CAD build for the part. Positions are in the model's coordinates, mm. Face numbers are marked on the shaded views. A direction names the side the tool comes from. Coordinates: 2 decimals unless noted, no trailing zeros. Loops run counter-clockwise (first coordinate to the right, second up) from the corner with the lowest first, then second, coordinate; pieces in that order, holes last. Notation, with made-up numbers: (-2, 69.25) - (38, 69.25) arc R30 cw to (38, 102.25) - close; hole circle Ø6 at (44, 6). An arc over 180 degrees is marked (long way). Put each result on its own line as item: value.
```python
from build123d import *

# Parameters (mm, degrees)
SALIENTE_EXTRUIR1_DEPTH    = 14
CROQUIS2_W                 = 0.4
CROQUIS2_H                 = 0.4
CORTAR_EXTRUIR1_DEPTH      = 1
CORTAR_EXTRUIR1_DEPTH_BACK = 15
SALIENTE_EXTRUIR2_DEPTH    = 14
CORTAR_EXTRUIR2_DEPTH      = 1
CORTAR_EXTRUIR2_DEPTH_BACK = 5.5
CORTAR_EXTRUIR3_DEPTH      = 5.5
SALIENTE_EXTRUIR3_DEPTH    = 14
CROQUIS7_R                 = 1
CORTAR_EXTRUIR4_DEPTH      = 4
REDONDEO3_R                = 0.4
CROQUIS9_R                 = 1
CORTAR_EXTRUIR5_DEPTH      = 18.5


with BuildPart() as part:
    # Croquis1 → Saliente-Extruir1 (new body)
    with BuildSketch(Plane.XY):
        with BuildLine():
            Line((0.5, 6.982120022), (0.5, 12.967496998))
            Line((0.5, 12.967496998), (3.5, 12.967496998))
            Line((3.5, 12.967496998), (3.5, 9.367496998))
            ThreePointArc((3.5, 9.367496998), (8.215838363, 5.700877125), (10, 0))
            Line((10, 0), (10, -11.6))
            ThreePointArc((10, -11.6), (10.117157288, -11.882842712), (10.4, -12))
            Line((10.4, -12), (14, -12))
            Line((14, -12), (14, -15))
            Line((14, -15), (7, -15))
            Line((7, -15), (7, -7.141428429))
            ThreePointArc((7, -7.141428429), (0, -10), (-7, -7.141428429))
            Line((-7, -7.141428429), (-7, -15))
            Line((-7, -15), (-14, -15))
            Line((-14, -15), (-14, -12))
            Line((-14, -12), (-10.4, -12))
            ThreePointArc((-10.4, -12), (-10.117157288, -11.882842712), (-10, -11.6))
            Line((-10, -11.6), (-10, 0))
            ThreePointArc((-10, 0), (-8.215838363, 5.700877125), (-3.5, 9.367496998))
            Line((-3.5, 9.367496998), (-3.5, 12.967496998))
            Line((-3.5, 12.967496998), (-0.5, 12.967496998))
            Line((-0.5, 12.967496998), (-0.5, 6.982120022))
            ThreePointArc((-0.5, 6.982120022), (0, -7), (0.5, 6.982120022))
        make_face()
    extrude(amount=SALIENTE_EXTRUIR1_DEPTH)

    # Croquis2 → Cortar-Extruir1 (cut, two sides)
    with BuildSketch(Plane.XY.offset(14)) as cortar_extruir1_sk:
        with Locations((-7.2, -14.8)):
            Rectangle(CROQUIS2_W, CROQUIS2_H)
        with Locations((7.2, -14.8)):
            Rectangle(CROQUIS2_W, CROQUIS2_H)
    extrude(amount=CORTAR_EXTRUIR1_DEPTH, mode=Mode.SUBTRACT)
    extrude(cortar_extruir1_sk.sketch, amount=-CORTAR_EXTRUIR1_DEPTH_BACK, mode=Mode.SUBTRACT)

    # Croquis4 → Saliente-Extruir2 (add, through all)
    with BuildSketch(Plane.XY.offset(14)):
        Polygon((-14, -12), (-10, 0), (-10, -12), align=None)
        Polygon((14, -12), (10, 0), (10, -12), align=None)
    extrude(amount=-SALIENTE_EXTRUIR2_DEPTH)

    # Croquis5 → Cortar-Extruir2 (cut, two sides)
    with BuildSketch(Plane.XY.offset(14)) as cortar_extruir2_sk:
        Polygon((-14, -12), (-10, 0), (-10, -12), align=None)
        Polygon((14, -12), (10, 0), (10, -12), align=None)
    extrude(amount=CORTAR_EXTRUIR2_DEPTH, mode=Mode.SUBTRACT)
    extrude(cortar_extruir2_sk.sketch, amount=-CORTAR_EXTRUIR2_DEPTH_BACK, mode=Mode.SUBTRACT)

    # Croquis6 → Cortar-Extruir3 (cut)
    with BuildSketch(Plane(origin=(0, 0, 0), x_dir=(-1, 0, 0), z_dir=(0, 0, -1))):
        Polygon((-14, -12), (-10, 0), (-10, -12), align=None)
        Polygon((14, -12), (10, 0), (10, -12), align=None)
    extrude(amount=-CORTAR_EXTRUIR3_DEPTH, mode=Mode.SUBTRACT)

    # Croquis1<2> → Saliente-Extruir3 (add, through all)
    with BuildSketch(Plane.XY):
        with BuildLine():
            Line((0.5, 6.982120022), (0.5, 12.967496998))
            Line((0.5, 12.967496998), (3.5, 12.967496998))
            Line((3.5, 12.967496998), (3.5, 9.367496998))
            ThreePointArc((3.5, 9.367496998), (8.215838363, 5.700877125), (10, 0))
            Line((10, 0), (10, -11.6))
            ThreePointArc((10, -11.6), (10.117157288, -11.882842712), (10.4, -12))
            Line((10.4, -12), (14, -12))
            Line((14, -12), (14, -15))
            Line((14, -15), (7, -15))
            Line((7, -15), (7, -7.141428429))
            ThreePointArc((7, -7.141428429), (0, -10), (-7, -7.141428429))
            Line((-7, -7.141428429), (-7, -15))
            Line((-7, -15), (-14, -15))
            Line((-14, -15), (-14, -12))
            Line((-14, -12), (-10.4, -12))
            ThreePointArc((-10.4, -12), (-10.117157288, -11.882842712), (-10, -11.6))
            Line((-10, -11.6), (-10, 0))
            ThreePointArc((-10, 0), (-8.215838363, 5.700877125), (-3.5, 9.367496998))
            Line((-3.5, 9.367496998), (-3.5, 12.967496998))
            Line((-3.5, 12.967496998), (-0.5, 12.967496998))
            Line((-0.5, 12.967496998), (-0.5, 6.982120022))
            ThreePointArc((-0.5, 6.982120022), (0, -7), (0.5, 6.982120022))
        make_face()
    extrude(amount=SALIENTE_EXTRUIR3_DEPTH)

    # Croquis7 → Cortar-Extruir4 (cut, through all)
    with BuildSketch(Plane(origin=(0, -12, 0), x_dir=(1, 0, 0), z_dir=(0, 1, 0))):
        with Locations((-12, -11.25)):
            Circle(CROQUIS7_R)
        with Locations((-12, -2.75)):
            Circle(CROQUIS7_R)
        with Locations((12, -2.75)):
            Circle(CROQUIS7_R)
        with Locations((12, -11.25)):
            Circle(CROQUIS7_R)
    extrude(amount=-CORTAR_EXTRUIR4_DEPTH, mode=Mode.SUBTRACT)

    # Redondeo3
    redondeo3_edges = [part.edges().sort_by_distance(p)[0] for p in [
        (-2, 12.967496998, 0),
        (2, 12.967496998, 14),
        (-2, 12.967496998, 14),
        (2, 12.967496998, 0),
    ]]
    fillet(redondeo3_edges, radius=REDONDEO3_R)

    # Croquis9 → Cortar-Extruir5 (cut, through all)
    with BuildSketch(Plane.ZY.offset(3.5)):
        with Locations((2.8, 11.167496998)):
            Circle(CROQUIS9_R)
        with Locations((7.000061, 11.167496998)):
            Circle(CROQUIS9_R)
        with Locations((11.200061, 11.167496998)):
            Circle(CROQUIS9_R)
    extrude(amount=-CORTAR_EXTRUIR5_DEPTH, mode=Mode.SUBTRACT)


solid = part.part
```
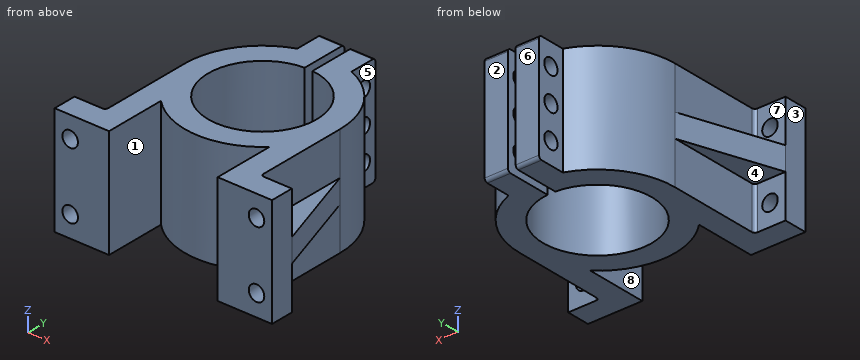
Q1. Wall check: L1, parallel to Z at x = -12, y = -14.05; L2, parallel to Y at x = -3, z = 2.5; L3, parallel to Y at x = 2.55, z = 2.8. Give the ranges that are in metal, low to high. Write a range as from..to.
Determined:
L1: 0..1.75, 3.75..10.25, 12.25..14
L2: -9.54..-6.32, 6.32..10.21, 12.12..12.97
L3: -9.67..-6.52, 6.52..10.17, 12.17..12.97
Q2. Tool access for the marked faces 4, 5, 6, 7 and 8: list every direction of +Z, -Z, +X, -X, +Y, -Y with a clear straight run to the whole face (end or side of a thin tool).
Determined:
face 4: -Z, -X, +Y
face 5: +Z, -Z, +X, +Y
face 6: +Z, -Z, +X, -X, +Y
face 7: +Z, -X, +Y
face 8: +Z, -Z, -Y
Q3. Slice it at B-B, the plane z = 7. Give the cut face in (x, y).
Determined:
outline: (-14, -15) - (-7, -15) - (-7, -7.14) arc R10 ccw to (7, -7.14) - (7, -15) - (14, -15) - (14, -12) - (10, 0) arc R10 ccw to (3.5, 9.37) - (3.5, 10.17) - (0.5, 10.17) - (0.5, 6.98) arc R7 cw (long way) to (-0.5, 6.98) - (-0.5, 10.17) - (-3.5, 10.17) - (-3.5, 9.37) arc R10 ccw to (-10, 0) - (-14, -12) - close; (-3.5, 12.17) - (-0.5, 12.17) - (-0.5, 12.97) - (-3.5, 12.97) - close; (0.5, 12.17) - (3.5, 12.17) - (3.5, 12.97) - (0.5, 12.97) - close
Q4. Mould opens along X. For the marked faces 1, 2 and 3 say: +X half, -X half, draft (parallel to the pull), parting line (faces both ways), or undercut.
Determined:
face 1: undercut
face 2: draft
face 3: -X half
Q5. Slice it at A-A, the plane x = -1.5. Give the cut face in (y, z), then the cut area to 3 significant figures.
Determined:
outline: (-9.89, 0) - (-6.84, 0) - (-6.84, 14) - (-9.89, 14) - close; (6.84, 0) - (12.57, 0) arc R0.4 ccw to (12.97, 0.4) - (12.97, 13.6) arc R0.4 ccw to (12.57, 14) - (6.84, 14) - close; hole circle Ø2 at (11.17, 2.8); hole circle Ø2 at (11.17, 7); hole circle Ø2 at (11.17, 11.2)
area: 119 mm2
Q6. Pin check, flat tips, straight feed: pin 1 Ø3 at (y, z) = (11.5, 6) entering from +X; pin 2 Ø8 at (y, z) = (10, 3.5) entering from +X; pin 3 Ø1.2 at (x, z) = (-12, 11.25) entering from +Y; pin 4 Ø1.6 at (y, z) = (-4, 2.5) entering from -X. Stop position of each tip, or through.
Determined:
pin 1: x = 3.5
pin 2: x = 8
pin 3: through
pin 4: x = -10
Q7. Slice it at C-C, the plane y = 2.75. Give the cut face in (x, z), then the cut area to 3 significant figures.
Determined:
outline: (-9.61, 0) - (-6.44, 0) - (-6.44, 14) - (-9.61, 14) - close; (6.44, 0) - (9.61, 0) - (9.61, 14) - (6.44, 14) - close
area: 89.0 mm2
Q8. Slice it at D-D, the plane x = 12. Give the cut face in (y, z).
Determined:
outline: (-15, 0) - (-12, 0) - (-12, 1.75) - (-15, 1.75) - close; (-15, 3.75) - (-12, 3.75) - (-12, 5.5) - (-6, 5.5) - (-6, 8.5) - (-12, 8.5) - (-12, 10.25) - (-15, 10.25) - close; (-15, 12.25) - (-12, 12.25) - (-12, 14) - (-15, 14) - close
